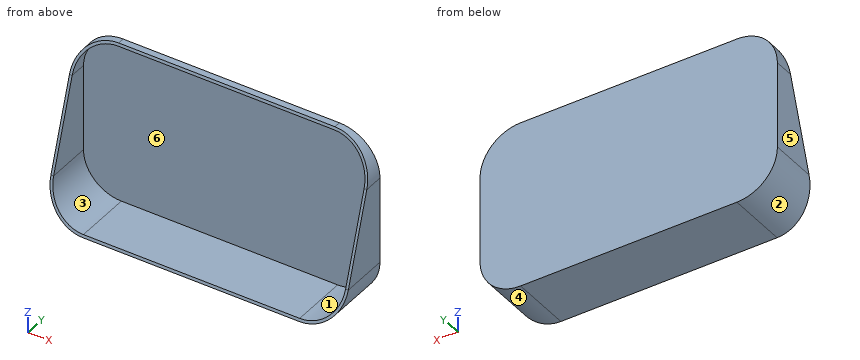
from build123d import *

# Parameters (mm, degrees)
BOSS_EXTRUDE1_DEPTH = 45
CUT_EXTRUDE2_DEPTH  = 43
CUT_EXTRUDE4_DEPTH  = 264


with BuildPart() as part:
    # Sketch1 → Boss-Extrude1 (new body)
    with BuildSketch(Plane(origin=(0, 0, 0), x_dir=(1, 0, 0), z_dir=(0, 1, 0))):
        with BuildLine():
            Line((-80, 62), (80, 62))
            ThreePointArc((80, 62), (101.213203436, 53.213203436), (110, 32))
            Line((110, 32), (110, -32))
            ThreePointArc((110, -32), (101.213203436, -53.213203436), (80, -62))
            Line((80, -62), (-80, -62))
            ThreePointArc((-80, -62), (-101.213203436, -53.213203436), (-110, -32))
            Line((-110, -32), (-110, 32))
            ThreePointArc((-110, 32), (-101.213203436, 53.213203436), (-80, 62))
        make_face()
    extrude(amount=BOSS_EXTRUDE1_DEPTH)

    # Sketch6 → Cut-Extrude2 (cut)
    with BuildSketch(Plane.XZ):
        with BuildLine():
            Line((80, 60), (-80, 60))
            ThreePointArc((-80, 60), (-99.798989873, 51.798989873), (-108, 32))
            Line((-108, 32), (-108, -32))
            ThreePointArc((-108, -32), (-99.798989873, -51.798989873), (-80, -60))
            Line((-80, -60), (80, -60))
            ThreePointArc((80, -60), (99.798989873, -51.798989873), (108, -32))
            Line((108, -32), (108, 32))
            ThreePointArc((108, 32), (99.798989873, 51.798989873), (80, 60))
        make_face()
    extrude(amount=-CUT_EXTRUDE2_DEPTH, mode=Mode.SUBTRACT)

    # Sketch4 → Cut-Extrude4 (cut)
    with BuildSketch(Plane(origin=(110, 0, 0), x_dir=(0, 0, -1), z_dir=(1, 0, 0))):
        Polygon((-32, 30.322580645), (-62, 40), (-62, 0), (-32, 0), align=None)
        Polygon((32, 9.677419355), (-32, 30.322580645), (-32, 0), (32, 0), align=None)
        Polygon((62, 0), (32, 9.677419355), (32, 0), align=None)
    extrude(amount=-CUT_EXTRUDE4_DEPTH, mode=Mode.SUBTRACT)


solid = part.part
Can you work these out from the model? Positions are in its coordinate system, mm. Face numbers are marked on the shaded views. A direction names the side the tool comes from. Coordinates: 2 decimals unless noted, no trailing zeros. Write each loop counter-clockwise with the first axis right and the second up, starting at its lowest first coordinate (ties: lowest second). Pieces come first, ordered by that corner, then holes.
Q1. Imagine slicing it at C-C, the plane z = 43. List the corners of the cut face in (x, y) for me, plus the area to 3 significant figures.
Results found:
outline: (-107.91, 33.87) - (-105.75, 33.87) - (-105.75, 43) - (105.75, 43) - (105.75, 33.87) - (107.91, 33.87) - (107.91, 45) - (-107.91, 45) - close
area: 471 mm2
Q2. Imagine slicing it at A-A, the plane y = 13. List the corners of the cut face in (x, z) for me.
Results found:
outline: (-110, -32) arc R30 ccw to (-80, -62) - (80, -62) arc R30 ccw to (110, -32) - (110, -21.7) - (108, -21.7) - (108, -32) arc R28 cw to (80, -60) - (-80, -60) arc R28 cw to (-108, -32) - (-108, -21.7) - (-110, -21.7) - close
Q3. Imagine slicing it at D-D, the plane y = 33.5. List the corners of the cut face in (x, z) for me, plus the area to 3 significant figures.
Results found:
outline: (-110, -32) arc R30 ccw to (-80, -62) - (80, -62) arc R30 ccw to (110, -32) - (110, 32) arc R30 ccw to (108.34, 41.85) - (106.21, 41.85) arc R28 cw to (108, 32) - (108, -32) arc R28 cw to (80, -60) - (-80, -60) arc R28 cw to (-108, -32) - (-108, 32) arc R28 cw to (-106.21, 41.85) - (-108.34, 41.85) arc R30 ccw to (-110, 32) - close
area: 798 mm2
Q4. If we mould it in two halves opening along X, with no side actions, what happens to the marked faces 1, 2, 3 and 4? For each: +X half, -X half, draft (parallel to the pull), parting line (faces both ways), or undercut.
Results found:
face 1: undercut
face 2: -X half
face 3: undercut
face 4: +X half
Q5. Imagine slicing it at B-B, the plane x = 45. List the corners of the cut face in (y, z) for me, plus the area to 3 significant figures.
Results found:
outline: (0, -62) - (45, -62) - (45, 62) - (40, 62) - (39.35, 60) - (43, 60) - (43, -60) - (0.65, -60) - close
area: 340 mm2
Q6. Which directions (+Z, -Z, +X, -X, +Y, -Y) give clear straight access to the entire face, cutting with the end or side of a thin tool? Please do the marked faces 5 and 6.
Results found:
face 5: +Z, -Z, -X, +Y, -Y
face 6: -Y
Q7. For P1, Ø4, axis at y = 10, z = -36, coming from the -X side; P2, Ø8, axis at y = 20.5, z = -37, coming from the +X side; P3, Ø10, axis at x = 43, y = 7.5, coming from the +Z side, each with a flat end and sliding along its axis, tell me the tip position at first contact or that it passes through.
Results found:
P1: stops at x = -109.93
P2: stops at x = 109.98
P3: stops at z = -60
Q8. Please list where these lines run through material, in increasing order: L1, parallel to X at y = 39.5, z = 30; L2, parallel to Z at x = -59, y = 40.5; L3, parallel to Y at x = -73.5, z = 43.
Results found:
L1: x = -110 to -108, 108 to 110
L2: z = -62 to -60, 60 to 62
L3: y = 43 to 45
